Part model, mm, in its own coordinate system. A direction names the side the tool comes from. Give positions to 0.01 mm unless a question says otherwise; leave off trailing zeros. Write each loop counter-clockwise with the first axis right and the second up, starting at its lowest first coordinate (ties: lowest second). Pieces come first, ordered by that corner, then holes. Notation, with made-up numbers: M 19,61 L 38,61 A22 ccw 38,88 Z; hole C 85,73.5 d3. An arc over 180 degrees is marked long. Write item = value, one per line. Start each with the question number.
from build123d import *

# Parameters (mm, degrees)
F0_W          = 50.8
F0_H          = 12.7
F1_DEPTH      = 12.7
F6_R          = 9.525
F7_ANGLE_BACK = 30
F7_ANGLE      = 60
F9_DEPTH      = 25.4
F10_W         = 12.827
F10_H         = 3.302
F11_DEPTH     = 25.4


with BuildPart() as f1:
    # F0 (on Top) → F1 (new body)
    with BuildSketch(Plane.XY):
        with Locations((25.4, 6.35)):
            Rectangle(F0_W, F0_H)
    extrude(amount=F1_DEPTH)

    # F6 (on 3pt) → F7 (revolve, cut)
    with BuildSketch(Plane(origin=(0, 6.35, 0), x_dir=(-1, 0, 0), z_dir=(0, 1, 0)), mode=Mode.PRIVATE) as f7_sk:
        with Locations((0, 6.35)):
            Circle(F6_R)
    revolve(f7_sk.sketch.rotate(Axis((25.4, 6.35, 6.3316160813), (0, 0, 1)), -F7_ANGLE_BACK), axis=Axis((25.4, 6.35, 6.3316160813), (0, 0, 1)), revolution_arc=F7_ANGLE, mode=Mode.SUBTRACT)

    # F8 (on face) → F9 (cut)
    with BuildSketch(Plane(origin=(0, 12.7, 0), x_dir=(-1, 0, 0), z_dir=(0, 1, 0))):
        with BuildLine():
            ThreePointArc((-50.8, 6.35), (-48.9401280605, 10.8401280605), (-44.45, 12.7))
            Line((-44.45, 12.7), (-50.8, 12.7))
            Line((-50.8, 12.7), (-50.8, 6.35))
        make_face()
        with BuildLine():
            ThreePointArc((-44.45, 0), (-48.9401280605, 1.8598719395), (-50.8, 6.35))
            Line((-50.8, 6.35), (-50.8, 0))
            Line((-50.8, 0), (-44.45, 0))
        make_face()
    extrude(amount=-F9_DEPTH, mode=Mode.SUBTRACT)

    # F10 (on face) → F11 (cut)
    with BuildSketch(Plane.XY.offset(12.7)):
        with Locations((44.3865, 4.7349631403)):
            Rectangle(F10_W, F10_H)
        with Locations((44.3865, 8.0369631403)):
            Rectangle(F10_W, F10_H)
    extrude(amount=-F11_DEPTH, mode=Mode.SUBTRACT)


solid = f1.part
Q1. Tool access for faces 1 (the face through (26, 6, 0)), 2 (the face through (44, 3.084, 6)): list every direction of +Z, -Z, +X, -X, +Y, -Y with a clear straight run to the whole face (end or side of a thin tool).
Q2. Slice it at A-A (x = 44). Give the cut face in (y, z).
Q3. Drop flat-ended pins along their axis: P1, Ø1, axis at x = 42.5, y = 9, coming from the -Z side; P2, Ø2, axis at y = 6, z = 3.5, coming from the +X side; P3, Ø3, axis at y = 11, z = 3, coming from the +X side. Give the stop position or say it passes through.
Q4. Slice it at B-B (z = 8.5). Give the cut face in (x, y).
Q5. Slice it at C-C (z = 5.75). Give the cut face in (x, y).
Q6. Probe line 1 along Y through (x, z) = (48, 8.5); line 2 along X through (y, z) = (7.5, 1.25); line 3 along X through (y, z) = (9.75, 11). List the from-to ranges inside material, lowest first.
Q7. Two-plate mould, pull along Y, no slides. Class faces 3 (the face through (29, 12.7, 6)), 4 (the face through (44, 9.688, 6)), 5 (the face through (26, 6, 12.7)), 6 (the face through (29, 0, 6)): +Y half, -Y half, draft (parallel to the pull), parting line (faces both ways), or undercut.
Working result:
q1.face_1 = -Z, +X, -X, +Y, -Y
q1.face_2 = +Z, -Z, +X
q2.outline = M 0,0 L 3.08,0 L 3.08,12.7 L 0,12.7 Z; M 9.69,0 L 12.7,0 L 12.7,12.7 L 9.69,12.7 Z
q3.P1 = through
q3.P2 = 37.97
q3.P3 = 50.52
q4.outline = M 10.58,0 L 50.42,0 L 50.42,3.08 L 37.97,3.08 L 37.97,9.69 L 50.42,9.69 L 50.42,12.7 L 10.58,12.7 A16.12 ccw Z
q5.outline = M 10.83,0 L 50.77,0 L 50.77,3.08 L 37.97,3.08 L 37.97,9.69 L 50.77,9.69 L 50.77,12.7 L 10.83,12.7 A15.89 ccw Z
q6.line_1 = 0 to 3.08, 9.69 to 12.7
q6.line_2 = 8.08 to 37.97
q6.line_3 = 8.65 to 48.77
q7.face_3 = +Y half
q7.face_4 = undercut
q7.face_5 = draft
q7.face_6 = -Y half
